Can you work these out from the model? Positions are in its coordinate system, mm. A direction names the side the tool comes from. Coordinates: 2 decimals unless noted, no trailing zeros. Loops run counter-clockwise (first coordinate to the right, second up) from the corner with the lowest first, then second, coordinate; pieces in that order, holes last. Notation, with made-up numbers: (75.5, -24) - (116.5, -24) arc R25 cw to (116.5, 15) - close; hole circle Ø4 at (85, 30.5). An arc over 180 degrees is marked (long way). Put each result on its own line as item: value. Start each with the question number.
from build123d import *

# Parameters (mm, degrees)
F0_R     = 4.7625
F1_DEPTH = 36.5125
F2_W     = 7.0995158286
F2_H     = 1.5875
F3_DEPTH = 7.9375
F4_W     = 7.0995158286
F4_H     = 1.5875
F5_DEPTH = 7.9375
F6_R     = 2.15265
F7_DEPTH = 8.9375001002


with BuildPart() as f1:
    # F0 (on Top) → F1 (new body)
    with BuildSketch(Plane.XY):
        Circle(F0_R)
    extrude(amount=F1_DEPTH)

    # F2 (on face) → F3 (cut)
    with BuildSketch(Plane.XY.offset(36.5125)):
        with Locations((0, -3.96875)):
            Rectangle(F2_W, F2_H)
    extrude(amount=-F3_DEPTH, mode=Mode.SUBTRACT)

    # F4 (on face) → F5 (cut)
    with BuildSketch(Plane(origin=(0, 0, 0), x_dir=(1, 0, 0), z_dir=(0, 0, -1))):
        with Locations((0, 3.96875)):
            Rectangle(F4_W, F4_H)
    extrude(amount=-F5_DEPTH, mode=Mode.SUBTRACT)

    # F6 (on face) → F7 (cut, up to face)
    with BuildSketch(Plane.XZ.offset(3.175)):
        with Locations((0, 32.54375)):
            Circle(F6_R)
        with Locations((0, 3.96875)):
            Circle(F6_R)
    extrude(amount=-F7_DEPTH, mode=Mode.SUBTRACT)


solid = f1.part
Q1. We'd pull the mould along Z, two halves only. Please class faces 1 (the flat face through (-2, -3.175, 6)), 2 (the flat face through (0, 1, 36.512)), 3 (the cylindrical face through (2.05, 0.74, 4.62)): released by +Z, released by -Z, zero draft, split by the parting line, or undercut.
Q2. Will these pins go through, and if not, where does the flat tip stop? pin 1 (4 mm diameter, centred on x = 3.5, z = 29, fed in from +Y); pin 2 (4 mm diameter, centred on x = 3.5, z = 10, fed in from -Y); pin 3 (5 mm diameter, centred on x = -3.5, z = 13, fed in from -Y).
Q3. I want a section at B-B on z = 5. List the corners of the cut face in (x, y) for me (1 decimal), and give its area (3 significant figures).
Q4. I want a section at C-C on z = 9. List the corners of the cut face in (x, y) for me (1 decimal).
Q5. Please list where these lines run through material, in increasing order: line 1 along Z through (x, y) = (0, 2.75); line 2 along Z through (x, y) = (-0.5, 3); line 3 along X through (y, z) = (0, 4). Write a range as [from, to].
Q6. I want a section at D-D on x = -1.5. List the corners of the cut face in (y, z) for me (1 decimal).
Q7. On a 3-axis mill with a long thin cutter (end or side, diameter ignored), from which of +Z, -Z, +X, -X, +Y, -Y can I reach the whole of each face in a straight line? I mean faces 4 (the flat face through (-2, -3.175, 34)), 5 (the flat face through (0, 1, 0)), 6 (the flat face through (0, -4, 7.938)). Say none if no direction works.
Q8. I want a section at A-A on x = 0. List the corners of the cut face in (y, z) for me (1 decimal).
Calculated:
1. face 1: zero draft
1. face 2: released by +Z
1. face 3: undercut
2. pin 1: y = 4.52
2. pin 2: y = -4.52
2. pin 3: y = -4.66
3. outline: (-3.5, -3.2) - (-1.9, -3.2) - (-1.9, 4.4) arc R4.8 ccw to start; (1.9, -3.2) - (3.5, -3.2) arc R4.8 ccw to (1.9, 4.4) - close
3. area: 33.9 mm2
4. outline: circle Ø9.5 at (0, 0)
5. line 1: [0, 1.82], [6.12, 30.39], [34.7, 36.51]
5. line 2: [0, 1.87], [6.06, 30.45], [34.64, 36.51]
5. line 3: [-4.76, -2.15], [2.15, 4.76]
6. outline: (-4.5, 7.9) - (-3.2, 7.9) - (-3.2, 5.5) - (4.5, 5.5) - (4.5, 31) - (-3.2, 31) - (-3.2, 28.6) - (-4.5, 28.6) - close; (-3.2, 0) - (4.5, 0) - (4.5, 2.4) - (-3.2, 2.4) - close; (-3.2, 34.1) - (4.5, 34.1) - (4.5, 36.5) - (-3.2, 36.5) - close
7. face 4: +Z, +X, -X, -Y
7. face 5: -Z, +X, -X, +Y, -Y
7. face 6: -Z, +X, -X, -Y
8. outline: (-4.8, 7.9) - (-3.2, 7.9) - (-3.2, 6.1) - (4.8, 6.1) - (4.8, 30.4) - (-3.2, 30.4) - (-3.2, 28.6) - (-4.8, 28.6) - close; (-3.2, 0) - (4.8, 0) - (4.8, 1.8) - (-3.2, 1.8) - close; (-3.2, 34.7) - (4.8, 34.7) - (4.8, 36.5) - (-3.2, 36.5) - close
